CAD build for the part. Positions are in the model's coordinates, mm. A direction names the side the tool comes from. Round coordinates to 2 decimals unless told otherwise and drop trailing zeros. Loops run counter-clockwise (first coordinate to the right, second up) from the corner with the lowest first, then second, coordinate; pieces in that order, holes last.
from build123d import *

# Parameters (mm, degrees)
SKETCH1_W           = 75
SKETCH1_H           = 30
BOSS_EXTRUDE1_DEPTH = 15
FILLET1_R           = 15
SKETCH2_W           = 45
SKETCH2_H           = 8
BOSS_EXTRUDE2_DEPTH = 45
FILLET2_R           = 5
FILLET3_R           = 3
SKETCH3_R           = 8
CUT_EXTRUDE1_DEPTH  = 2


with BuildPart() as part:
    # Sketch1 → Boss-Extrude1 (new body)
    with BuildSketch(Plane.XY):
        with Locations((-40, 23.52978815)):
            Rectangle(SKETCH1_W, SKETCH1_H)
    extrude(amount=-BOSS_EXTRUDE1_DEPTH)

    # Fillet1
    fillet1_edges = [part.edges().sort_by_distance(p)[0] for p in [
        (-77.5, 8.52978815, -7.5),
        (-77.5, 38.52978815, -7.5),
        (-2.5, 8.52978815, -7.5),
        (-2.5, 38.52978815, -7.5),
    ]]
    fillet(fillet1_edges, radius=FILLET1_R - 0.0001)  # a hair under: the kernel refuses the full size

    # Sketch2 → Boss-Extrude2 (add)
    with BuildSketch(Plane(origin=(0, 0, -15), x_dir=(-1, 0, 0), z_dir=(0, 0, -1))):
        with Locations((40, 19.52978815)):
            Rectangle(SKETCH2_W, SKETCH2_H)
    extrude(amount=BOSS_EXTRUDE2_DEPTH)

    # Fillet2
    fillet2_edges = [part.edges().sort_by_distance(p)[0] for p in [
        (-62.5, 19.52978815, -60),
        (-17.5, 19.52978815, -60),
    ]]
    fillet(fillet2_edges, radius=FILLET2_R)

    # Fillet3
    fillet3_edges = [part.edges().sort_by_distance(p)[0] for p in [
        (-40, 8.52978815, 0),
        (-40, 38.52978815, 0),
        (-6.893368993, 34.136419158, 0),
        (-6.893368993, 12.923157143, 0),
        (-73.106631007, 34.136419158, 0),
        (-73.106631007, 12.923157143, 0),
        (-40, 8.52978815, -15),
        (-40, 38.52978815, -15),
        (-6.893368993, 34.136419158, -15),
        (-6.893368993, 12.923157143, -15),
        (-73.106631007, 34.136419158, -15),
        (-73.106631007, 12.923157143, -15),
    ]]
    fillet(fillet3_edges, radius=FILLET3_R)

    # Sketch3 → Cut-Extrude1 (cut)
    with BuildSketch(Plane.XY):
        with Locations((-58.148379701, 23.52978815)):
            Circle(SKETCH3_R)
    extrude(amount=-CUT_EXTRUDE1_DEPTH, mode=Mode.SUBTRACT)


solid = part.part
Item 1: Mould opens along X. For faces 4 (the cylindrical face through (-61.07, 19.59, -58.5)), 5 (the flat face through (-17.5, 19, -35)), 6 (the flat face through (-40, 23.53, -37)), 7 (the cylindrical face through (-50.758, 20.466, -0.986)) say: released by +X, released by -X, zero draft, split by the parting line, or undercut.
Verdict:
face 4: released by -X
face 5: released by +X
face 6: zero draft
face 7: undercut
Item 2: Wall check: L1, parallel to Y at x = -45, z = -36; L2, parallel to Z at x = -37.5, y = 12; L3, parallel to X at y = 23, z = -53. Give the ranges that are in metal, low to high.
Verdict:
L1: y = 15.53 to 23.53
L2: z = -15 to 0
L3: x = -62.5 to -17.5
Item 3: 3-axis set-ups, long thin cutter, end or side, ignore diameter. For faces 1 (the flat face through (-62.5, 19, -35)), 2 (the flat face through (-40, 24, 0)), 3 (the flat face through (-58, 24, -2)): which of +Z, -Z, +X, -X, +Y, -Y reach the whole face in a straight line?
Verdict:
face 1: -Z, -X, +Y, -Y
face 2: +Z, +X, -X, +Y, -Y
face 3: +Z
Item 4: Cut at C-C (z = -39). List the corners of the cut face in (x, y), plus the area to 3 significant figures.
Verdict:
outline: (-62.5, 15.53) - (-17.5, 15.53) - (-17.5, 23.53) - (-62.5, 23.53) - close
area: 360 mm2
Item 5: Flat gauge pins, fed straight in: P1, Ø6, axis at x = -58.5, z = -46.5, coming from the -Y side; P2, Ø5, axis at x = -60.5, y = 26.5, coming from the +Z side; P3, Ø5, axis at x = -61, z = -43, coming from the +Y side. Where does each tip first touch, or does it go through?
Verdict:
P1: stops at y = 15.53
P2: stops at z = -2
P3: stops at y = 23.53
Item 6: Cut at B-B (x = -29.5). List the corners of the cut face in (y, z).
Verdict:
outline: (8.53, -12) arc R3 ccw to (11.53, -15) - (15.53, -15) - (15.53, -60) - (23.53, -60) - (23.53, -15) - (35.53, -15) arc R3 ccw to (38.53, -12) - (38.53, -3) arc R3 ccw to (35.53, 0) - (11.53, 0) arc R3 ccw to (8.53, -3) - close
